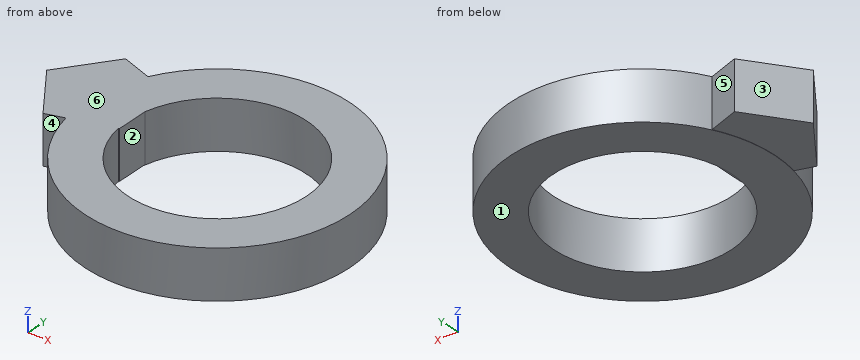
```python
from build123d import *

# Parameters (mm, degrees)
F3_R     = 68.807709
F3_R_2   = 46.350216
F1_DEPTH = 25.4
F4_DEPTH = 25.194961


with BuildPart() as f1:
    # F3 (on face) → F1 (new body)
    with BuildSketch(Plane.XY):
        Circle(F3_R)
        Circle(F3_R_2, mode=Mode.SUBTRACT)
    extrude(amount=F1_DEPTH)

    # F2 (on face) → F4 (join)
    with BuildSketch(Plane.XY.offset(25.4)):
        Polygon((-45.300776, -6.761135), (-45.300776, 26.375637), (-76.815719, 36.615463), (-96.293024, 9.807251), (-76.815719, -17.00096), align=None)
    extrude(amount=-F4_DEPTH)


solid = f1.part
```
Here's how the part is built. I have some questions about the finished solid (model axes, mm). Face numbers are marked on the shaded views. A direction names the side the tool comes from. Give positions to 0.01 mm unless a question says otherwise; leave off trailing zeros. Loops run counter-clockwise (first coordinate to the right, second up) from the corner with the lowest first, then second, coordinate; pieces in that order, holes last. Notation, with made-up numbers: M -40,-1.75 L 5,-1.75 A20 ccw 5,19.25 Z; hole C 62,-28 d4. An arc over 180 degrees is marked long. Return JSON: item names as keys, results as strings.
Item 1: Imagine slicing it at C-C on y = -35. List the corners of the cut face in (x, z) for me, then the cut area to 3 significant figures.
A:
{"outline": "M -59.24,0 L -30.39,0 L -30.39,25.4 L -59.24,25.4 Z; M 30.39,0 L 59.24,0 L 59.24,25.4 L 30.39,25.4 Z", "area": "1,470 mm^2"}
Item 2: I'm going to push flat-ended pins straight in: pin 1 Ø1 at (y, z) = (-2.5, 3.5) entering from -X; pin 2 Ø4 at (x, z) = (-55, 15) entering from +Y; pin 3 Ø1.5 at (x, z) = (-31, 6.5) entering from -Y. Where does each tip first touch, or does it pass through?
A:
{"pin 1": "stops at x = -87.71", "pin 2": "stops at y = 43.88", "pin 3": "stops at y = -61.8"}
Item 3: Thinking about a two-plate mould opening in X: for the marked faces 1, 2 and 3, which applies, released by +X, released by -X, zero draft, split by the parting line, or undercut?
A:
{"face 1": "zero draft", "face 2": "undercut", "face 3": "released by -X"}
Item 4: Imagine slicing it at D-D on y = 0. List the corners of the cut face in (x, z) for me, then the cut area to 3 significant figures.
A:
{"outline": "M -89.17,0.21 L -68.81,0.21 L -68.81,0 L -46.35,0 L -46.35,0.21 L -45.3,0.21 L -45.3,25.4 L -89.17,25.4 Z; M 46.35,0 L 68.81,0 L 68.81,25.4 L 46.35,25.4 Z", "area": "1,680 mm^2"}
Item 5: Imagine slicing it at B-B on z = 7. List the corners of the cut face in (x, y) for me.
A:
{"outline": "M -96.29,9.81 L -76.82,-17 L -67.38,-13.94 A68.81 ccw long -61.16,31.53 L -76.82,36.62 Z; hole M -45.83,-6.93 A46.35 ccw long -45.3,9.81 L -45.3,-6.76 Z"}
Item 6: Imagine slicing it at A-A on x = 0. List the corners of the cut face in (y, z) for me.
A:
{"outline": "M -68.81,0 L -46.35,0 L -46.35,25.4 L -68.81,25.4 Z; M 46.35,0 L 68.81,0 L 68.81,25.4 L 46.35,25.4 Z"}
Item 7: On a 3-axis mill with a long thin cutter (end or side, diameter ignored), from which of +Z, -Z, +X, -X, +Y, -Y can I reach the whole of each face in a straight line? I mean the marked faces 4, 5 and 6. Say none if no direction works.
A:
{"face 4": "+Z, -Z, -Y", "face 5": "+Z, -Z, +Y", "face 6": "+Z, +X, -X, +Y, -Y"}
Item 8: Please list where these lines run through material, in increasing order: line 1 (Y direction, x = 0, z = 20); line 2 (Y direction, x = -36, z = 12); line 3 (X direction, y = -32, z = 12.25).
A:
{"line 1": "y = -68.81 to -46.35, 46.35 to 68.81", "line 2": "y = -58.64 to -29.19, 29.19 to 58.64", "line 3": "x = -60.91 to -33.53, 33.53 to 60.91"}
